Could you check a few things on this model? Use its own coordinates, in mm. Round coordinates to 2 decimals unless told otherwise and drop trailing zeros. Loops run counter-clockwise (first coordinate to the right, second up) from the corner with the lowest first, then second, coordinate; pieces in that order, holes last. Notation, with made-up numbers: M -25,86.25 L -20,86.25 A15 cw -20,105.25 Z; hole C 42.5,84.25 d3. An arc over 180 degrees is marked long. One line per item, written item: value. Start each with the question number.
Q1. Imagine slicing it at B-B (y = 0). Please give me the cut outline in (x, z), then the cut area to 3 significant figures.
Q2. Imagine slicing it at C-C (z = 0). Please give me the cut outline in (x, y), then the cut area to 3 significant figures.
Q3. I'm going to push flat-ended pins straight in: pin 1 Ø13 at (y, z) = (0, 0) entering from -X; pin 2 Ø2 at (x, z) = (4.5, 94) entering from -Y; pin 3 Ø1 at (x, y) = (3.5, -26.5) entering from +Z; pin 4 Ø3 at (x, y) = (4.5, 4.5) entering from -Z. Where does each tip first touch, or does it pass through?
Q4. Imagine slicing it at A-A (x = 2). Please give me the cut outline in (y, z) (3 decimals).
Q5. Please list where these lines run through material, in increasing order: line 1 along Y through (x, z) = (2.7, 0); line 2 along Y through (x, z) = (1.3, 280); line 3 along Z through (x, y) = (0.5, -15).
Q6. Imagine slicing it at D-D (z = 162). Please give me the cut outline in (x, y).
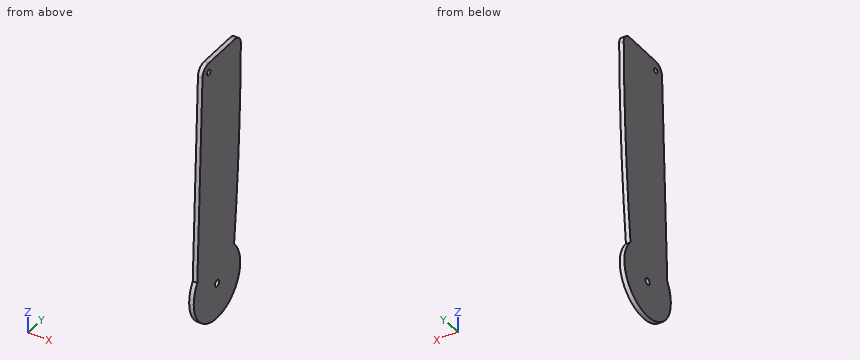
from build123d import *

# Parameters (mm, degrees)
SKETCH2_R           = 4
SKETCH2_R_2         = 3.175
BOSS_EXTRUDE1_DEPTH = 5.588


with BuildPart() as part:
    # Sketch2 → Boss-Extrude1 (new body)
    with BuildSketch(Plane(origin=(0, 0, 0), x_dir=(0, 0, -1), z_dir=(1, 0, 0))):
        with BuildLine():
            Line((-292, 33.638045694), (-292, -15.648345659))
            ThreePointArc((-292, -15.648345659), (-288.648466484, -23.967241468), (-280.46599542, -27.639294256))
            Line((-280.46599542, -27.639294256), (-23.677807257, -37.618664829))
            ThreePointArc((-23.677807257, -37.618664829), (44.264265693, 4.059221924), (-30.124927866, 32.684724583))
            ThreePointArc((-30.124927866, 32.684724583), (-154.873072642, 41.908750383), (-279.906177735, 45.637678913))
            ThreePointArc((-279.906177735, 45.637678913), (-288.452045102, 42.156433663), (-292, 33.638045694))
        make_face()
        Circle(SKETCH2_R, mode=Mode.SUBTRACT)
        with Locations((-280, -15.648345659)):
            Circle(SKETCH2_R_2, mode=Mode.SUBTRACT)
    extrude(amount=BOSS_EXTRUDE1_DEPTH)


solid = part.part
Report:
1. outline: M 0,-44.45 L 5.59,-44.45 L 5.59,-4 L 0,-4 Z; M 0,4 L 5.59,4 L 5.59,292 L 0,292 Z
1. area: 1,840 mm²
2. outline: M 0,-44.45 L 5.59,-44.45 L 5.59,-4 L 0,-4 Z; M 0,4 L 5.59,4 L 5.59,44.45 L 0,44.45 Z
2. area: 452 mm²
3. pin 1: stops at x = 0
3. pin 2: stops at y = -34.92
3. pin 3: stops at z = 286.07
3. pin 4: stops at z = -44.35
4. outline: M -37.619,23.678 A44.45 ccw long 32.685,30.125 A2843.66 ccw 45.638,279.906 A12 ccw 33.638,292 L -15.648,292 A12 ccw -27.639,280.466 Z; hole C -15.648,280 d6.35; hole C 0,0 d8
5. line 1: y = -44.45 to -4, 4 to 44.45
5. line 2: y = -27.66 to -18.82, -12.47 to 45.64
5. line 3: z = -41.84 to 276.89, 283.11 to 292
6. outline: M 0,-32.24 L 5.59,-32.24 L 5.59,42.27 L 0,42.27 Z
